Can you work these out from the model? Positions are in its coordinate system, mm. A direction names the side the tool comes from. Give positions to 0.01 mm unless a question says otherwise; leave off trailing zeros. Loops run counter-clockwise (first coordinate to the right, second up) from the corner with the lowest first, then second, coordinate; pieces in that order, holes last. Notation, with made-up numbers: M 13.5,43.25 L 60.5,43.25 A8 cw 60.5,55.25 Z; hole C -28,-39 d9. An arc over 180 degrees is marked long. Put each result on its own line as item: value. Start each with the question number.
1) For P1, Ø3, axis at x = 18, y = 4.5, coming from the +Z side; P2, Ø12, axis at x = 7, y = -32.5, coming from the -Z side; P3, Ø5, axis at x = -9, y = -25, coming from the +Z side; P4, Ø6, axis at x = 21.5, y = -14, coming from the +Z side, each with a flat end and sliding along its axis, tell me the tip position at first contact or that it passes through.
2) Imagine slicing it at D-D (z = 25). Write out the boundary of the cut face in (x, y).
3) Imagine slicing it at B-B (x = 8). Write out the boundary of the cut face in (y, z), then the cut area to 3 significant figures.
4) For faces 4 (the flat face through (-2, -32, 1)), 5 (the cylindrical face through (15.931, 6.764, 3.986)), 6 (the flat face through (0, -24, 30)), which set-ups out of +Z, -Z, +X, -X, +Y, -Y let a thin tool reach every point of the face, with its end or its side?
5) Imagine slicing it at A-A (z = 15). Write out the boundary of the cut face in (x, y), then the cut area to 3 significant figures.
6) If we mould it in two halves opening along Y, with no side actions, what happens to faces 1 (the flat face through (38, -16, 30)), 2 (the flat face through (36, -15, 24)), 3 (the cylindrical face through (19.59, 4.67, 14.37))? For each: +Y half, -Y half, draft (parallel to the pull), parting line (faces both ways), or undercut.
7) Please list where these lines run through material, in increasing order: line 1 along Y through (x, z) = (0, 28.7); line 2 along Y through (x, z) = (0, 2); line 3 along Y through (x, z) = (15.5, 22.5). Write a range as from..to.
8) Imagine slicing it at C-C (y = 0). Write out the boundary of the cut face in (x, z), then the cut area to 3 significant figures.
from build123d import *

# Parameters (mm, degrees)
SKETCH_1_R              = 42.5
SKETCH_1_R_2            = 40.5
EXTRUDE_1_DEPTH         = 30
SKETCH_2_R              = 40.5
SKETCH_2_R_2            = 38.5
EXTRUDE_2_DEPTH         = 24
EXTRUDE_3_OUTLINE_R     = 38.5
EXTRUDE_3_DEPTH         = 3
SKETCH_5_R              = 1.75
EXTRUDE_4_DEPTH         = 27
SKETCH_10_R             = 3
EXTRUDE_10_DEPTH        = 1.5
SKETCH_21_R             = 1.5
CUT_EXTRUDE_1_DEPTH     = 66.289738857
SKETCH_6_R              = 1.5
EXTRUDE_5_DEPTH         = 28
SKETCH_7_R              = 3
EXTRUDE_6_DEPTH         = 2
SKETCH_8_R              = 1.45
EXTRUDE_7_DEPTH         = 21
SKETCH_9_R              = 3
EXTRUDE_8_DEPTH         = 2
SKETCH_22_R             = 2.5
CUT_EXTRUDE_2_DEPTH     = 1
SKETCH_23_R             = 1.5
EXTRUDE_11_DEPTH        = 28
SKETCH_25_R             = 3
EXTRUDE_12_DEPTH        = 5
CUT_EXTRUDE_START       = -40.635067554
CUT_EXTRUDE_3_OUTLINE_R = 4
CUT_EXTRUDE_3_DEPTH     = 8.016303225


# Read off the part's stored shape, not the designer's step: 凸台-拉伸3, 切除-拉伸3
with BuildPart() as part:
    # 草图1 → 凸台-拉伸1 (new body)
    with BuildSketch(Plane.XY):
        Circle(SKETCH_1_R)
        Circle(SKETCH_1_R_2, mode=Mode.SUBTRACT)
    extrude(amount=EXTRUDE_1_DEPTH)

    # 草图2 → 凸台-拉伸2 (add)
    with BuildSketch(Plane.XY):
        Circle(SKETCH_2_R)
        Circle(SKETCH_2_R_2, mode=Mode.SUBTRACT)
    extrude(amount=EXTRUDE_2_DEPTH)

    # 凸台-拉伸3 outline → 凸台-拉伸3 (add)
    with BuildSketch(Plane.XY):
        Circle(EXTRUDE_3_OUTLINE_R)
    extrude(amount=EXTRUDE_3_DEPTH)

    # 草图5 → 凸台-拉伸4 (add)
    with BuildSketch(Plane.XY.offset(3)):
        with Locations((0, -24)):
            Circle(SKETCH_5_R)
    extrude(amount=EXTRUDE_4_DEPTH)

    # 草图10 → 凸台-拉伸10 (add)
    with BuildSketch(Plane.XY.offset(3)):
        with Locations((8, -24)):
            Circle(SKETCH_10_R)
        with Locations((0, -16)):
            Circle(SKETCH_10_R)
        with Locations((-8, -24)):
            Circle(SKETCH_10_R)
        with Locations((0, -32)):
            Circle(SKETCH_10_R)
    extrude(amount=EXTRUDE_10_DEPTH)

    # 草图21 → 切除-拉伸1 (cut, through all)
    with BuildSketch(Plane.XY.offset(4.5)):
        with Locations((-8, -24)):
            Circle(SKETCH_21_R)
        with Locations((0, -16)):
            Circle(SKETCH_21_R)
        with Locations((8, -24)):
            Circle(SKETCH_21_R)
        with Locations((0, -32)):
            Circle(SKETCH_21_R)
    extrude(amount=-CUT_EXTRUDE_1_DEPTH, mode=Mode.SUBTRACT)

    # 草图6 → 凸台-拉伸5 (add)
    with BuildSketch(Plane.XY.offset(3)):
        with Locations((15.773694335, -13.86328125)):
            Circle(SKETCH_6_R)
    extrude(amount=EXTRUDE_5_DEPTH)

    # 草图7 → 凸台-拉伸6 (add)
    with BuildSketch(Plane.XY.offset(3)):
        with Locations((15.773694335, -13.86328125)):
            Circle(SKETCH_7_R)
    extrude(amount=EXTRUDE_6_DEPTH)

    # 草图8 → 凸台-拉伸7 (add)
    with BuildSketch(Plane.XY.offset(3)):
        with Locations(Location((18.141870405, 4.736563967, 0), (0, 0, 180))):
            Circle(SKETCH_8_R)
    extrude(amount=EXTRUDE_7_DEPTH)

    # 草图9 → 凸台-拉伸8 (add)
    with BuildSketch(Plane.XY.offset(3)):
        with Locations((18.141870405, 4.736563967)):
            Circle(SKETCH_9_R)
    extrude(amount=EXTRUDE_8_DEPTH)

    # 草图22 → 切除-拉伸2 (cut)
    with BuildSketch(Plane(origin=(0, 0, 0), x_dir=(-1, 0, 0), z_dir=(0, 0, -1))):
        with Locations((-8, -24)):
            Circle(SKETCH_22_R)
        with Locations((0, -16)):
            Circle(SKETCH_22_R)
        with Locations((8, -24)):
            Circle(SKETCH_22_R)
        with Locations((0, -32)):
            Circle(SKETCH_22_R)
    extrude(amount=-CUT_EXTRUDE_2_DEPTH, mode=Mode.SUBTRACT)

    # 草图23 → 凸台-拉伸11 (add)
    with BuildSketch(Plane.XY.offset(3)):
        Circle(SKETCH_23_R)
    extrude(amount=EXTRUDE_11_DEPTH)

    # 草图25 → 凸台-拉伸12 (add)
    with BuildSketch(Plane.XY.offset(3)):
        Circle(SKETCH_25_R)
    extrude(amount=EXTRUDE_12_DEPTH)

    # 切除-拉伸3 outline → 切除-拉伸3 (cut)
    with BuildSketch(Plane(origin=(0, 0, 0), x_dir=(0.707106781186546, -0.707106781186549, 0), z_dir=(0.707106781186549, 0.707106781186546, 0)).offset(CUT_EXTRUDE_START)):
        with Locations((16.451557856, -7.167019764)):
            Circle(CUT_EXTRUDE_3_OUTLINE_R)
    extrude(amount=CUT_EXTRUDE_3_DEPTH, mode=Mode.SUBTRACT)


solid = part.part
Recorded:
1. P1: z = 24
1. P2: z = 0
1. P3: z = 4.5
1. P4: z = 5
2. outline: C 0,0 d85; C 0,-24 d3.5; C 0,0 d3; C 15.77,-13.86 d3; hole C 0,0 d81
3. outline: M -41.74,0 L -26.5,0 L -26.5,1 L -25.5,1 L -25.5,4.5 L -27,4.5 L -27,3 L -37.66,3 L -37.66,24 L -39.7,24 L -39.7,30 L -41.74,30 Z; M -22.5,1 L -21.5,1 L -21.5,0 L 41.74,0 L 41.74,30 L 39.7,30 L 39.7,24 L 37.66,24 L 37.66,3 L -21,3 L -21,4.5 L -22.5,4.5 Z
3. area: 440 mm²
4. face 4: -Z
4. face 5: +Z
4. face 6: +Z, +X, -X, -Y
5. outline: C 0,0 d85; C 0,-24 d3.5; C 0,0 d3; C 15.77,-13.86 d3; C 18.14,4.74 d2.9; hole C 0,0 d77
5. area: 1,050 mm²
6. face 1: draft
6. face 2: undercut
6. face 3: undercut
7. line 1: -42.5..-40.5, -25.75..-22.25, -1.5..1.5, 40.5..42.5
7. line 2: -42.5..-33.5, -30.5..-17.5, -14.5..42.5
7. line 3: -39.57..-35.24, -15.34..-12.39, 35.24..39.57
8. outline: M -42.5,0 L 42.5,0 L 42.5,30 L 40.5,30 L 40.5,24 L 38.5,24 L 38.5,3 L 3,3 L 3,8 L 1.5,8 L 1.5,31 L -1.5,31 L -1.5,8 L -3,8 L -3,3 L -38.5,3 L -38.5,24 L -40.5,24 L -40.5,30 L -42.5,30 Z
8. area: 546 mm²
